Here's the drawing with two shaded views (mm, measured from the low corner). I have some questions. A direction names the side the tool comes from. Round coordinates to 2 decimals unless told otherwise and drop trailing zeros. Order: outer loops, then holes, each group sorted by start corner. A loop starts at its lowest first (then second) coordinate and runs counter-clockwise, first axis right, second up. Notation, with made-up numbers: (45.25, -12) - (49.25, -12) arc R21 cw to (49.25, 3) - close; hole circle Ø1 at (74, 32.5). An arc over 180 degrees is marked (long way). One line per item, written item: value.
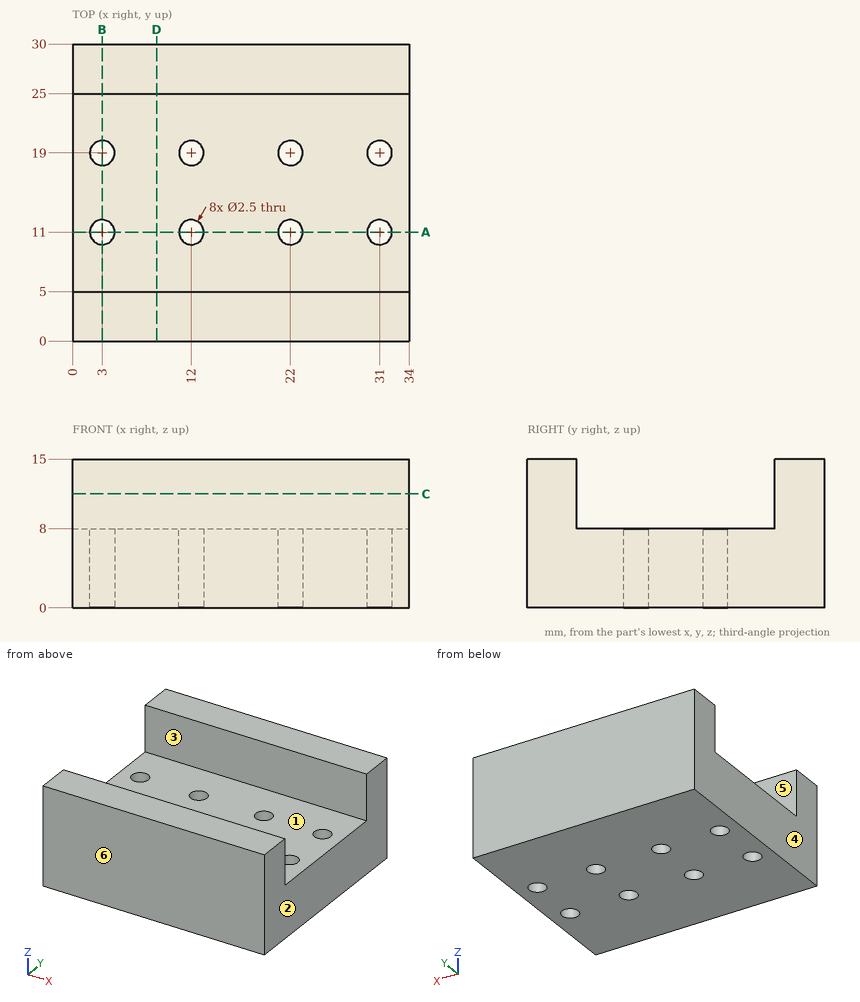
Q1. If we section it at B-B, the plane x = 3: Please give me the cut outline in (y, z), then the cut area to 3 significant figures.
Results list:
outline: (0, 0) - (9.75, 0) - (9.75, 8) - (5, 8) - (5, 15) - (0, 15) - close; (12.25, 0) - (17.75, 0) - (17.75, 8) - (12.25, 8) - close; (20.25, 0) - (30, 0) - (30, 15) - (25, 15) - (25, 8) - (20.25, 8) - close
area: 270 mm²
Q2. We'd pull the mould along Y, two halves only. Please class the marked faces 3, 4, 5 and 6: released by +Y, released by -Y, zero draft, split by the parting line, or undercut.
Results list:
face 3: undercut
face 4: zero draft
face 5: undercut
face 6: released by -Y
Q3. Will these pins go through, and if not, where does the flat tip stop? pin 1 (2 mm diameter, centred on x = 31, y = 11, fed in from +Z); pin 2 (6 mm diameter, centred on x = 15.5, y = 12, fed in from +Z).
Results list:
pin 1: through
pin 2: z = 8
Q4. If we section it at D-D, the plane x = 8.5: Please give me the cut outline in (y, z), then the cut area to 3 significant figures.
Results list:
outline: (0, 0) - (30, 0) - (30, 15) - (25, 15) - (25, 8) - (5, 8) - (5, 15) - (0, 15) - close
area: 310 mm²
Q5. If we section it at C-C, the plane z = 11.5: Please give me the cut outline in (x, y).
Results list:
outline: (0, 0) - (34, 0) - (34, 5) - (0, 5) - close; (0, 25) - (34, 25) - (34, 30) - (0, 30) - close
Q6. If I drill on line 1 along Y through (x, z) = (12, 2.5); line 2 along X through (y, z) = (11, 2); line 3 along Y through (x, z) = (30.5, 13.5), over which ranges is the centre line in solid material (lowest first)?
Results list:
line 1: 0 to 9.75, 12.25 to 17.75, 20.25 to 30
line 2: 0 to 1.75, 4.25 to 10.75, 13.25 to 20.75, 23.25 to 29.75, 32.25 to 34
line 3: 0 to 5, 25 to 30
Q7. Which directions (+Z, -Z, +X, -X, +Y, -Y) give clear straight access to the entire face, cutting with the end or side of a thin tool? Please do the marked faces 1 and 2.
Results list:
face 1: +Z, +X, -X
face 2: +Z, -Z, +X, +Y, -Y
Q8. If we section it at A-A, the plane y = 11: Please give me the cut outline in (x, z), then the cut area to 3 significant figures.
Results list:
outline: (0, 0) - (1.75, 0) - (1.75, 8) - (0, 8) - close; (4.25, 0) - (10.75, 0) - (10.75, 8) - (4.25, 8) - close; (13.25, 0) - (20.75, 0) - (20.75, 8) - (13.25, 8) - close; (23.25, 0) - (29.75, 0) - (29.75, 8) - (23.25, 8) - close; (32.25, 0) - (34, 0) - (34, 8) - (32.25, 8) - close
area: 192 mm²
